Build history of the part. All positions in model axes, mm. Face numbers are marked on the shaded views. A direction names the side the tool comes from. Round coordinates to 2 decimals unless told otherwise and drop trailing zeros. Write each loop counter-clockwise with the first axis right and the second up, starting at its lowest first coordinate (ties: lowest second). Pieces come first, ordered by that corner, then holes. Notation, with made-up numbers: (72, 68) -> (120, 68) arc R26 ccw to (120, 107) -> close; hole circle Ø5 at (3, 36). An arc over 180 degrees is marked (long way). Return JSON: item names as keys, results as strings.
from build123d import *

# Parameters (mm, degrees)
F0_W     = 8
F0_H     = 2.5
F0_W_2   = 3
F0_H_2   = 40
F1_DEPTH = 50
F2_R     = 5


with BuildPart() as f1:
    # F0 (on Top) → F1 (new body)
    with BuildSketch(Plane.XY):
        with Locations((16, 0)):
            Rectangle(F0_W, F0_H)
        Polygon((-12, 1.25), (-12, -1.25), (12, -1.25), (12, 1.25), (9, 1.25), (-9, 1.25), align=None)
        with Locations((-16, 0)):
            Rectangle(F0_W, F0_H)
        with Locations((10.5, 21.25)):
            Rectangle(F0_W_2, F0_H_2)
        with Locations((-10.5, 21.25)):
            Rectangle(F0_W_2, F0_H_2)
    extrude(amount=F1_DEPTH)

    # F2
    f2_edges = [f1.edges().sort_by_distance(p)[0] for p in [
        (12, 1.25, 25),
        (-12, 1.25, 25),
        (-9, 1.25, 25),
        (9, 1.25, 25),
    ]]
    fillet(f2_edges, radius=F2_R)


solid = f1.part
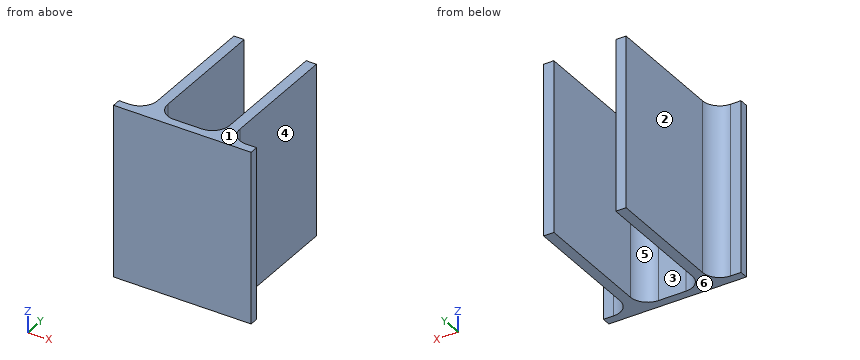
Q1. 3-axis set-ups, long thin cutter, end or side, ignore diameter. For the marked faces 1, 2 and 3: which of +Z, -Z, +X, -X, +Y, -Y reach the whole face in a straight line?
Verdict:
{"face 1": "+Z, +X, -X, +Y, -Y", "face 2": "+Z, -Z, -X, +Y", "face 3": "+Z, -Z, +Y"}
Q2. Saw through at A-A on y = 34.5. List the corners of the cut face in (x, z), then the cut area to 3 significant figures.
Verdict:
{"outline": "(-12, 0) -> (-9, 0) -> (-9, 50) -> (-12, 50) -> close; (9, 0) -> (12, 0) -> (12, 50) -> (9, 50) -> close", "area": "300 mm²"}
Q3. Wall check: L1, parallel to X at y = 35.5, z = 34; L2, parallel to Y at x = 0, z = 38; L3, parallel to X at y = 3, z = 5. Give the ranges that are in metal, low to high.
Verdict:
{"L1": "x = -12 to -9, 9 to 12", "L2": "y = -1.25 to 1.25", "L3": "x = -13.2 to -7.8, 7.8 to 13.2"}
Q4. Pin check, flat tips, straight feed: pin 1 Ø17.5 at (y, z) = (19, 29) entering from +X; pin 2 Ø10 at (y, z) = (27.5, 42) entering from -X; pin 3 Ø0.9 at (x, z) = (-19, 31.5) entering from +Y. Stop position of each tip, or through.
Verdict:
{"pin 1": "stops at x = 12", "pin 2": "stops at x = -12", "pin 3": "stops at y = 1.25"}
Q5. Saw through at D-D on x = 13.5. List the corners of the cut face in (y, z), then the cut area to 3 significant figures.
Verdict:
{"outline": "(-1.25, 0) -> (2.68, 0) -> (2.68, 50) -> (-1.25, 50) -> close", "area": "196 mm²"}
Q6. Two-plate mould, pull along X, no slides. Class the marked faces 4, 5 and 6: +X half, -X half, draft (parallel to the pull), parting line (faces both ways), or undercut.
Verdict:
{"face 4": "+X half", "face 5": "undercut", "face 6": "draft"}
Q7. Saw through at B-B on z = 11. List the corners of the cut face in (x, y), then the cut area to 3 significant figures.
Verdict:
{"outline": "(-20, -1.25) -> (20, -1.25) -> (20, 1.25) -> (17, 1.25) arc R5 cw to (12, 6.25) -> (12, 41.25) -> (9, 41.25) -> (9, 6.25) arc R5 cw to (4, 1.25) -> (-4, 1.25) arc R5 cw to (-9, 6.25) -> (-9, 41.25) -> (-12, 41.25) -> (-12, 6.25) arc R5 cw to (-17, 1.25) -> (-20, 1.25) -> close", "area": "361 mm²"}
Q8. Saw through at C-C on x = -1. List the corners of the cut face in (y, z), then the cut area to 3 significant figures.
Verdict:
{"outline": "(-1.25, 0) -> (1.25, 0) -> (1.25, 50) -> (-1.25, 50) -> close", "area": "125 mm²"}
